Can you work these out from the model? Positions are in its coordinate system, mm. A direction names the side the tool comes from. Round coordinates to 2 decimals unless told otherwise and drop trailing zeros. Loops run counter-clockwise (first coordinate to the right, second up) from the corner with the lowest first, then second, coordinate; pieces in that order, holes last.
(1) I want a section at A-A on z = -1. Write out the boundary of the cut face in (x, y).
(2) I want a section at B-B on y = -6.25. Write out the boundary of the cut face in (x, z).
(3) If I drill on line 1 along X through (y, z) = (-0.5, -5); line 2 along Y through (x, z) = (10.5, 0.25); line 3 along Z through (x, y) = (17.5, 7.75), over which ranges is the centre line in solid material (lowest first)?
(4) I want a section at C-C on x = 1.5. Write out the boundary of the cut face in (y, z).
(5) Which directions (+Z, -Z, +X, -X, +Y, -Y) give clear straight access to the entire face, cutting with the end or side of a thin tool? Please do faces 4 (the face through (19, 2.6, -1)), 5 (the face through (19.7, 0, -2)), 6 (the face through (-7, 0, 0.4)), 7 (the face through (-19.43, 0.11, 1.9)), 8 (the face through (19, -2.6, -1)).
(6) Thinking about a two-plate mould opening in Y: for faces 1 (the face through (-19.43, 9.4, 0.25)), 2 (the face through (-10.01, 2.25, -1.46)), 3 (the face through (10.016, -2.112, -4.782)), which applies, released by +Y, released by -Y, zero draft, split by the parting line, or undercut?
(7) Will these pins go through, and if not, where does the flat tip stop? pin 1 Ø0.5 at (y, z) = (-1.5, -1.5) entering from +X; pin 2 Ø0.5 at (y, z) = (-1.5, -4) entering from -X; pin 3 Ø1 at (x, y) = (-9.5, 5.5) entering from -Z; pin 4 Ø5 at (x, z) = (-2.5, -1) entering from -Y.
(8) I want a section at D-D on z = -4.5. Write out the boundary of the cut face in (x, y), plus the area to 3 significant figures.
from build123d import *

# Parameters (mm, degrees)
SKETCH1_W           = 40
SKETCH1_H           = 20
BOSS_EXTRUDE1_DEPTH = 2.5
FILLET1_R           = 2
SKETCH2_W           = 34
SKETCH2_H           = 14
CUT_EXTRUDE1_DEPTH  = 1
BOSS_EXTRUDE2_DEPTH = 2.6
FILLET2_R           = 1
BOSS_EXTRUDE3_DEPTH = 7
BOSS_EXTRUDE4_DEPTH = 0.6
LPATTERN1_COUNT     = 2
LPATTERN1_PITCH     = 20


with BuildPart() as part:
    # Sketch1 → Boss-Extrude1 (new body)
    with BuildSketch(Plane.XY):
        Rectangle(SKETCH1_W, SKETCH1_H)
    extrude(amount=BOSS_EXTRUDE1_DEPTH)

    # Fillet1
    fillet1_edges = [part.edges().sort_by_distance(p)[0] for p in [
        (20, 0, 2.5),
        (0, 10, 2.5),
        (-20, 0, 2.5),
        (0, -10, 2.5),
        (-20, 10, 1.25),
        (20, 10, 1.25),
        (20, -10, 1.25),
        (-20, -10, 1.25),
    ]]
    fillet(fillet1_edges, radius=FILLET1_R)

    # Sketch2 → Cut-Extrude1 (cut)
    with BuildSketch(Plane(origin=(0, 0, 0), x_dir=(-1, 0, 0), z_dir=(0, 0, -1))):
        Rectangle(SKETCH2_W, SKETCH2_H)
    extrude(amount=-CUT_EXTRUDE1_DEPTH, mode=Mode.SUBTRACT)

    # Sketch3 → Boss-Extrude2 (add, symmetric)
    with BuildSketch(Plane(origin=(0, 0, 0), x_dir=(0, 0, -1), z_dir=(0, 1, 0))):
        Polygon((0, -17), (3, -18.091910703), (3, -19.7), (0, -19.7), align=None)
    extrude(amount=BOSS_EXTRUDE2_DEPTH, both=True)

    # Fillet2
    fillet2_edges = [part.edges().sort_by_distance(p)[0] for p in [
        (18.895955351, -2.6, -3),
        (18.895955351, 2.6, -3),
    ]]
    fillet(fillet2_edges, radius=FILLET2_R)

    # Sketch4 → Boss-Extrude3 (add)
    with BuildSketch(Plane(origin=(0, 0, 1), x_dir=(-1, 0, 0), z_dir=(0, 0, -1))):
        with BuildLine():
            Line((-12.015564437, -1), (-11, -1))
            Line((-11, -1), (-11, -2.015564437))
            ThreePointArc((-11, -2.015564437), (-10, -2.25), (-9, -2.015564437))
            Line((-9, -2.015564437), (-9, -1))
            Line((-9, -1), (-7.984435563, -1))
            ThreePointArc((-7.984435563, -1), (-7.75, 0), (-7.984435563, 1))
            Line((-7.984435563, 1), (-9, 1))
            Line((-9, 1), (-9, 2.015564437))
            ThreePointArc((-9, 2.015564437), (-10, 2.25), (-11, 2.015564437))
            Line((-11, 2.015564437), (-11, 1))
            Line((-11, 1), (-12.015564437, 1))
            ThreePointArc((-12.015564437, 1), (-12.25, 0), (-12.015564437, -1))
        make_face()
    boss_extrude3 = extrude(amount=BOSS_EXTRUDE3_DEPTH)

    # Sketch5 → Cut-Revolve1 (revolve, cut)
    with BuildSketch(Plane(origin=(0, 0, 0), x_dir=(0, 0, -1), z_dir=(0, 1, 0))):
        with BuildLine():
            Line((4, -7.75), (6, -7.75))
            Line((6, -7.75), (6, -8.522203777))
            ThreePointArc((6, -8.522203777), (5.883022222, -8.200809972), (5.586824089, -8.0297999))
            Line((5.586824089, -8.0297999), (4, -7.75))
        make_face()
    cut_revolve1 = revolve(axis=Axis((10, 0, 1), (0, 0, -1)), mode=Mode.SUBTRACT)

    # Sketch6 → Boss-Extrude4 (add)
    with BuildSketch(Plane(origin=(0, 0, 1), x_dir=(-1, 0, 0), z_dir=(0, 0, -1))):
        with BuildLine():
            Line((-13.354101966, -1), (-6.645898034, -1))
            ThreePointArc((-6.645898034, -1), (-6.5, 0), (-6.645898034, 1))
            Line((-6.645898034, 1), (-13.354101966, 1))
            ThreePointArc((-13.354101966, 1), (-13.5, 0), (-13.354101966, -1))
        make_face()
    boss_extrude4 = extrude(amount=BOSS_EXTRUDE4_DEPTH)

    # LPattern1: Boss-Extrude3, Cut-Revolve1, Boss-Extrude4 ×2
    with Locations(*[(-i * LPATTERN1_PITCH, 0, 0) for i in range(1, LPATTERN1_COUNT)]):
        add(boss_extrude3)
        add(cut_revolve1, mode=Mode.SUBTRACT)
        add(boss_extrude4)


solid = part.part
Filled sheet:
1. outline: (-12.02, -1) - (-11, -1) - (-11, -2.02) arc R2.25 ccw to (-9, -2.02) - (-9, -1) - (-7.98, -1) arc R2.25 ccw to (-7.98, 1) - (-9, 1) - (-9, 2.02) arc R2.25 ccw to (-11, 2.02) - (-11, 1) - (-12.02, 1) arc R2.25 ccw to start; (7.98, -1) - (9, -1) - (9, -2.02) arc R2.25 ccw to (11, -2.02) - (11, -1) - (12.02, -1) arc R2.25 ccw to (12.02, 1) - (11, 1) - (11, 2.02) arc R2.25 ccw to (9, 2.02) - (9, 1) - (7.98, 1) arc R2.25 ccw to start; (17.36, -2.6) - (19.7, -2.6) - (19.7, 2.6) - (17.36, 2.6) - close
2. outline: (-20, 0) - (-17, 0) - (-17, 1) - (17, 1) - (17, 0) - (20, 0) - (20, 0.5) arc R2 ccw to (18, 2.5) - (-18, 2.5) arc R2 ccw to (-20, 0.5) - close
3. line 1: x = -12.01 to -7.99, 7.99 to 12.01
3. line 2: y = -10 to -7, -2.19 to 2.19, 7 to 10
3. line 3: z = 0 to 2.5
4. outline: (-10, 0) - (-7, 0) - (-7, 1) - (7, 1) - (7, 0) - (10, 0) - (10, 0.5) arc R2 ccw to (8, 2.5) - (-8, 2.5) arc R2 ccw to (-10, 0.5) - close
5. face 4: -Z, +X, -X, +Y
5. face 5: -Z, +X, +Y, -Y
5. face 6: -Z
5. face 7: +Z, -X, +Y, -Y
5. face 8: -Z, +X, -X, -Y
6. face 1: released by +Y
6. face 2: undercut
6. face 3: released by -Y
7. pin 1: stops at x = 19.7
7. pin 2: stops at x = -11
7. pin 3: stops at z = 1
7. pin 4: stops at y = -10
8. outline: (-11.92, -1) - (-11, -1) - (-11, -1.92) arc R2.16 ccw to (-9, -1.92) - (-9, -1) - (-8.08, -1) arc R2.16 ccw to (-8.08, 1) - (-9, 1) - (-9, 1.92) arc R2.16 ccw to (-11, 1.92) - (-11, 1) - (-11.92, 1) arc R2.16 ccw to start; (8.08, -1) - (9, -1) - (9, -1.92) arc R2.16 ccw to (11, -1.92) - (11, -1) - (11.92, -1) arc R2.16 ccw to (11.92, 1) - (11, 1) - (11, 1.92) arc R2.16 ccw to (9, 1.92) - (9, 1) - (8.08, 1) arc R2.16 ccw to start
8. area: 25.3 mm2
